Autodesk Inventor part; units mm, degrees
ref_plane "YZ Plane" through (0, 0, 0) normal (1, 0, 0) x (0, 1, 0)
ref_plane "XZ Plane" through (0, 0, 0) normal (0, 1, 0) x (-1, 0, 0)
ref_plane "XY Plane" through (0, 0, 0) normal (0, 0, 1) x (1, 0, 0)
sketch "Sketch1" plane through (0, 0, 0) normal (0, 1, 0) x (-1, 0, 0)
  line L0 (-107.95, -0.0035) -> (-53.978, 93.4857)
  line L1 (-53.978, 93.4857) -> (53.972, 93.4892)
  line L2 (53.972, 93.4892) -> (107.95, 0.0035)
  line L3 (107.95, 0.0035) -> (53.978, -93.4857)
  line L4 (53.978, -93.4857) -> (-53.972, -93.4892)
  line L5 (-53.972, -93.4892) -> (-107.95, -0.0035)
  line L6 (-92.964, 0.0336) -> (-46.4529, 80.526)
  line L7 (-46.4529, 80.526) -> (46.5111, 80.4924)
  line L8 (46.5111, 80.4924) -> (92.964, -0.0336)
  line L9 (92.964, -0.0336) -> (46.4529, -80.526)
  line L10 (46.4529, -80.526) -> (-46.5111, -80.4924)
  line L11 (-46.5111, -80.4924) -> (-92.964, 0.0336)
  line L12 (53.978, -93.4857) -> (46.4529, -80.526)
  line L13 (-53.972, -93.4892) -> (-46.5111, -80.4924)
  point P0 (0, 0)
  point P1 (0, 0)
  point P2 (0, 0)
  point P3 (0, 0)
  dimension "d0" = 215.9
  dimension "d1" = 14.986
extrude "Extrusion1" add sketch "Sketch1" along normal blind 107.95 contours L13 L10 L12 L4
sketch "Sketch2" plane through (46.5111, 0, -80.4924) normal (-0.0003616, 0, 0.9999999) x (0.9999999, 0, 0.0003616)
  line L0 (-92.9641, 0) -> (-92.9641, 107.95)
  line L1 (-92.9641, 107.95) -> (0, 107.95)
  line L2 (-92.9641, 0) -> (0, 0)
  line L3 (0, 0) -> (0, 107.95)
  line L4 (-73.9141, 88.9) -> (-19.05, 88.9)
  line L5 (-19.05, 88.9) -> (-19.05, 38.1)
  line L6 (-19.05, 38.1) -> (-73.9141, 38.1)
  line L7 (-73.9141, 38.1) -> (-73.9141, 88.9)
  point P0 (-46.482, 0)
  dimension "d4" = 19.05
  dimension "d5" = 19.05
  dimension "d6" = 38.1
  dimension "d7" = 19.05
extrude "Extrusion2" cut sketch "Sketch2" against normal up to surface (12.9965 mm away) contours L4 L5 L6 L7
sketch "Sketch3" plane through (53.972, 0, -93.4892) normal (-0.000032, 0, -1) x (-1, 0, 0.000032)
  line L0 (0, 107.95) -> (107.95, 107.95)
  line L1 (0, 0) -> (0, 107.95)
  line L2 (26.5062, 88.9) -> (81.3702, 88.9)
  line L3 (26.5062, 38.1) -> (26.5062, 88.9)
  line L4 (81.3702, 88.9) -> (81.3702, 38.1)
  line L5 (81.3702, 38.1) -> (26.5062, 38.1)
  line L6 (20.1562, 95.25) -> (87.7202, 95.25)
  line L7 (87.7202, 95.25) -> (87.7202, 31.75)
  line L8 (87.7202, 31.75) -> (20.1562, 31.75)
  line L9 (20.1562, 31.75) -> (20.1562, 95.25)
  point P0 (53.975, 0)
  dimension "d12" = 6.35
  dimension "d13" = 6.35
  dimension "d14" = 6.35
  dimension "d15" = 6.35
extrude "Extrusion3" cut sketch "Sketch3" against normal blind 3.175 contours L2 L4 L5 L3 | L6 L7 L8 L9
equation "\"d7\" = d4"
equation "\"d14\" = d13"
equation "\"d15\" = d12"
properties part number "SatelliteSideWallSensor_v2"
Read the model definition and answer for the solid it produces. Units are mm, in the model's axes. A direction names the side the tool comes from. Give positions to 0.01 mm unless a question says otherwise; leave off trailing zeros. Loops run counter-clockwise (first coordinate to the right, second up) from the corner with the lowest first, then second, coordinate; pieces in that order, holes last. Notation, with made-up numbers: (64.25, 88) -> (116.25, 88) arc R33 ccw to (116.25, 119) -> close; hole circle Ø8 at (-39.75, 3.5). An arc over 180 degrees is marked (long way). Use a Markdown table: item, result.
Q1. A tool of negligible diameter and unlimited length cuts with its end or side. For faces 1 (the face through (0, 88.9, -85)), 2 (the face through (-50.27, 53.22, -87.1)), 3 (the face through (1, 95.25, -92)), from which of +Z, -Z, +X, -X, +Y, -Y can it reach the whole face along a straight path? Write none if from no direction.
Solved:
| item | result |
|---|---|
| face 1 | +Z, -Z |
| face 2 | +Z, -X, +Y, -Y |
| face 3 | -Z |
Q2. Find the intervals of material crossed by line 1 along Y through (x, z) = (25, -84); line 2 along Y through (x, z) = (-31, -91.25); line 3 along Z through (x, y) = (-30, 55), in increasing order.
Solved:
| item | result |
|---|---|
| line 1 | y = 0 to 38.1, 88.9 to 107.95 |
| line 2 | y = 0 to 31.75, 95.25 to 107.95 |
| line 3 | z = -90.31 to -80.52 |
Q3. Section C-C, the plane z = -85.5 is taken. Determine the outline of the cut face in (x, y).
Solved:
| item | result |
|---|---|
| outline | (-49.34, 0) -> (49.39, 0) -> (49.39, 107.95) -> (-49.34, 107.95) -> close; hole (-27.4, 38.1) -> (27.46, 38.1) -> (27.46, 88.9) -> (-27.4, 88.9) -> close |
Q4. Section A-A, the plane y = 79.5 is taken. Determine the outline of the cut face in (x, z), then the cut area to 3 significant figures.
Solved:
| item | result |
|---|---|
| outline | (-53.98, -93.49) -> (-33.75, -93.49) -> (-33.75, -90.31) -> (-27.4, -90.31) -> (-27.4, -80.52) -> (-46.45, -80.53) -> close; (27.46, -90.31) -> (33.82, -90.31) -> (33.82, -93.49) -> (53.97, -93.49) -> (46.51, -80.49) -> (27.46, -80.5) -> close |
| area | 551 mm^2 |
Q5. Determine the mould class of faces 4 (the face through (1, 0, -87)), 5 (the face through (50.294, 53.219, -87.082)), 6 (the face through (1, 107.95, -87)), 7 (the face through (1, 92, -90.314)) for opening direction Y: pulls with the +Y half, pulls with the -Y half, needs draft (parallel to the pull), parting line crosses it, or undercut.
Solved:
| item | result |
|---|---|
| face 4 | pulls with the -Y half |
| face 5 | needs draft |
| face 6 | pulls with the +Y half |
| face 7 | undercut |
Q6. Each of these flat-tipped pins is pushed along its axis until it touches: pin 1 (5 mm diameter, centred on x = 30, y = 36, fed in from -Z); pin 2 (1.6 mm diameter, centred on y = 57.5, z = -91.5, fed in from +X); pin 3 (2.5 mm diameter, centred on y = 74, z = -92, fed in from -X). Where does it stop, or does it pass through?
Solved:
| item | result |
|---|---|
| pin 1 | stops at z = -90.31 |
| pin 2 | stops at x = 53.29 |
| pin 3 | stops at x = -53.84 |
Q7. Section D-D, the plane y = 14 is taken. Determine the outline of the cut face in (x, z).
Solved:
| item | result |
|---|---|
| outline | (-53.98, -93.49) -> (53.97, -93.49) -> (46.51, -80.49) -> (-46.45, -80.53) -> close |
Q8. Section B-B, the plane x = 17 is taken. Determine the outline of the cut face in (y, z).
Solved:
| item | result |
|---|---|
| outline | (0, -93.49) -> (31.75, -93.49) -> (31.75, -90.31) -> (38.1, -90.31) -> (38.1, -80.5) -> (0, -80.5) -> close; (88.9, -90.31) -> (95.25, -90.31) -> (95.25, -93.49) -> (107.95, -93.49) -> (107.95, -80.5) -> (88.9, -80.5) -> close |
